Part print with two shaded views. Sizes in mm from the minimum x, y, z corner. A direction names the side the tool comes from. Round coordinates to 2 decimals unless told otherwise and drop trailing zeros. Loops run counter-clockwise (first coordinate to the right, second up) from the corner with the lowest first, then second, coordinate; pieces in that order, holes last.
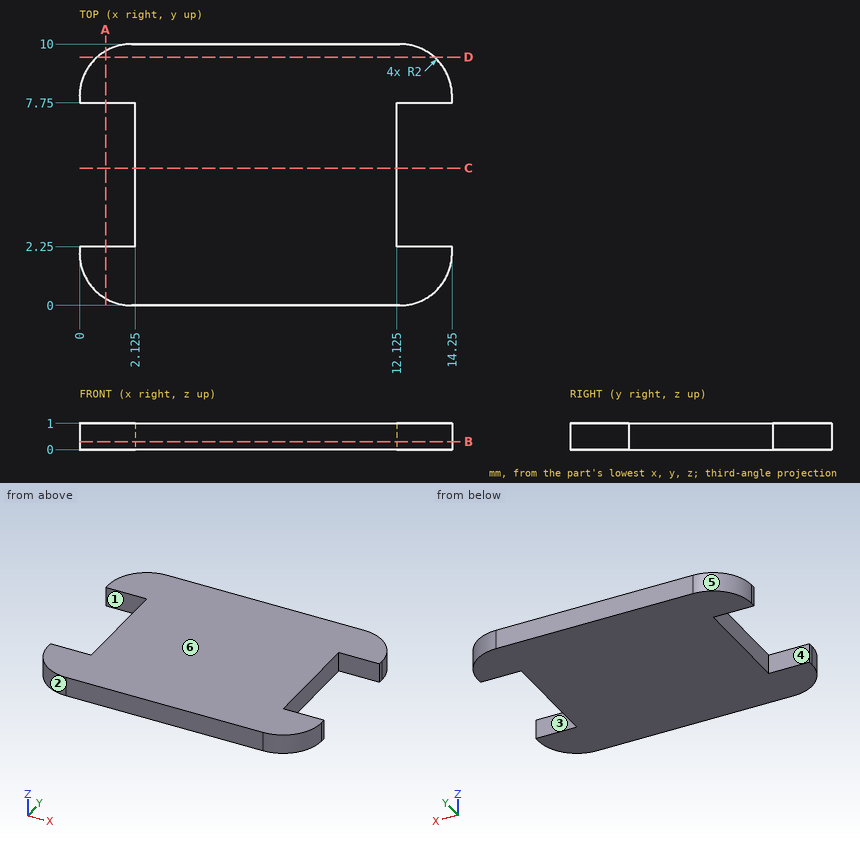
Item 1: Cut at A-A (x = 1). List the corners of the cut face in (y, z).
Verdict:
outline: (0.27, 0) - (2.25, 0) - (2.25, 1) - (0.27, 1) - close; (7.75, 0) - (9.73, 0) - (9.73, 1) - (7.75, 1) - close
Item 2: Wall check: L1, parallel to X at y = 3.25, z = 0.1 (3 decimals); L2, parallel to Y at x = 13.75, z = 0.55; L3, parallel to Y at x = 13.25, z = 0.3. Give the ranges that are in metal, low to high.
Verdict:
L1: x = 2.125 to 12.125
L2: y = 0.68 to 2.25, 7.75 to 9.32
L3: y = 0.27 to 2.25, 7.75 to 9.73
Item 3: 3-axis set-ups, long thin cutter, end or side, ignore diameter. For the marked faces 1, 2 and 3: which of +Z, -Z, +X, -X, +Y, -Y reach the whole face in a straight line?
Verdict:
face 1: +Z, -Z, -X
face 2: +Z, -Z, -X, -Y
face 3: +Z, -Z, +X
Item 4: Cut at C-C (y = 5.25). List the corners of the cut face in (x, z) (3 decimals), plus the area to 3 significant figures.
Verdict:
outline: (2.125, 0) - (12.125, 0) - (12.125, 1) - (2.125, 1) - close
area: 10.0 mm2
Item 5: Mould opens along Y. For the marked faces 4, 5 and 6 say: released by +Y, released by -Y, zero draft, split by the parting line, or undercut.
Verdict:
face 4: undercut
face 5: released by +Y
face 6: zero draft
Item 6: Flat gauge pins, fed straight in: P1, Ø0.5, axis at x = 1, z = 0.5, coming from the +Y side; P2, Ø3, axis at x = 12.5, y = 4, coming from the +Z side. Where does each tip first touch, or does it go through?
Verdict:
P1: stops at y = 9.85
P2: stops at z = 1
Item 7: Cut at D-D (y = 9.5). List the corners of the cut face in (x, z), plus the area to 3 significant figures.
Verdict:
outline: (0.68, 0) - (13.57, 0) - (13.57, 1) - (0.68, 1) - close
area: 12.9 mm2
Item 8: Cut at B-B (z = 0.3). List the corners of the cut face in (x, y) (3 decimals).
Verdict:
outline: (0, 2) arc R2 ccw to (2, 0) - (12.25, 0) arc R2 ccw to (14.25, 2) - (14.25, 2.25) - (12.125, 2.25) - (12.125, 7.75) - (14.25, 7.75) - (14.25, 8) arc R2 ccw to (12.25, 10) - (2, 10) arc R2 ccw to (0, 8) - (0, 7.75) - (2.125, 7.75) - (2.125, 2.25) - (0, 2.25) - close
